Geometry: final body of the model. Coordinates: model frame, mm. Face numbers are marked on the shaded views. Give positions to 0.01 mm unless a question says otherwise; leave off trailing zeros. Write each loop counter-clockwise with the first axis right and the second up, starting at its lowest first coordinate (ties: lowest second). Pieces come first, ordered by that corner, then holes.
Autodesk Inventor part; units mm, degrees
ref_plane "YZ Plane" through (0, 0, 0) normal (1, 0, 0) x (0, 1, 0)
ref_plane "XZ Plane" through (0, 0, 0) normal (0, 1, 0) x (-1, 0, 0)
ref_plane "XY Plane" through (0, 0, 0) normal (0, 0, 1) x (1, 0, 0)
sketch "Эскиз1" plane through (0, 0, 0) normal (0, 0, 1) x (1, 0, 0)
  line L0 (0, 14) -> (0, -14)
  line L1 (21, 14) -> (21.6, 14)
  line L2 (22, 13.6) -> (22, -13.6)
  line L3 (21.6, -14) -> (21, -14)
  line L4 (21, -14) -> (21, 14)
  line L5 (22, 13.6) -> (21.6, 14)
  line L6 (22, -13.6) -> (21.6, -14)
  point P0 (0, 0)
  point P1 (0, 0)
  point P2 (22, -14)
  point P3 (22, 14)
  dimension "d0" = 28
  dimension "d1" = 44
  dimension "d2" = 42
  dimension "d3" = 0.4
  dimension "d4" = 45
  dimension "d5" = 0.4
  dimension "d6" = 45
revolve "Вращение1" add sketch "Эскиз1" angle 360 about axis through (0, 14, 0) along (0, -1, 0)
sketch "Эскиз2" plane through (0, 0, 0) normal (0, 0, 1) x (1, 0, 0)
  circle A0 centre (0, 0) radius 5
  dimension "d8" = 10
extrude "Выдавливание1" cut sketch "Эскиз2" along normal through all both and the other way through all
equation "\"d6\" = d4"
properties part number "75. Втулка шестерни второй передачи"
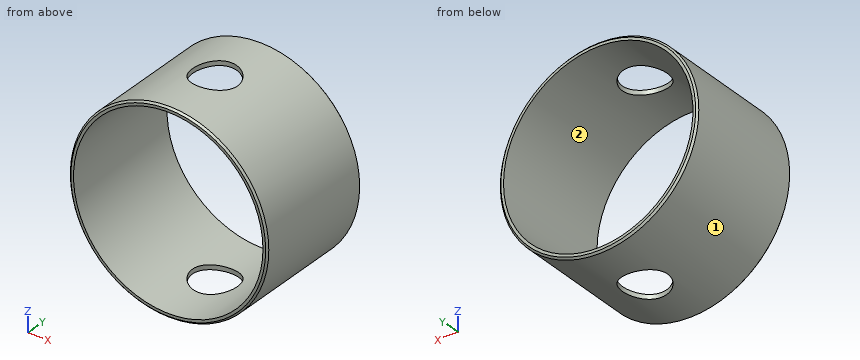
Q1. Section A-A on x = 0. Output: boundary loops of the cut face in (y, z), plus the area to 3 significant figures.
Filled sheet:
outline: (-14, -21.6) - (-13.6, -22) - (-5, -22) - (-5, -21) - (-14, -21) - close; (-14, 21) - (-5, 21) - (-5, 22) - (-13.6, 22) - (-14, 21.6) - close; (5, -22) - (13.6, -22) - (14, -21.6) - (14, -21) - (5, -21) - close; (5, 21) - (14, 21) - (14, 21.6) - (13.6, 22) - (5, 22) - close
area: 35.7 mm2
Q2. Pull-direction query (Z, two-part tool) for the marked faces 1 and 2; classes: released by +Z, released by -Z, zero draft, split by the parting line, or undercut.
Filled sheet:
face 1: split by the parting line
face 2: undercut
Q3. Section D-D on y = 6.5. Output: boundary loops of the cut face in (x, z), plus the area to 3 significant figures.
Filled sheet:
outline: circle Ø44 at (0, 0); hole circle Ø42 at (0, 0)
area: 135 mm2
Q4. Section B-B on z = 0. Output: boundary loops of the cut face in (x, y).
Filled sheet:
outline: (-22, -13.6) - (-21.6, -14) - (-21, -14) - (-21, 14) - (-21.6, 14) - (-22, 13.6) - close; (21, -14) - (21.6, -14) - (22, -13.6) - (22, 13.6) - (21.6, 14) - (21, 14) - close
Q5. Pin query (flat end, axial travel): P1, Ø5, axis at y = 4.5, z = 10, coming from the +X side; P2, Ø3, axis at x = -15, y = -3, coming from the +Z side; P3, Ø6, axis at x = 3.5, y = -3.5, coming from the +Z side. Return the tip coordinate at first contact, or that it passes through.
Filled sheet:
P1: stops at x = 20.68
P2: stops at z = 17.37
P3: stops at z = 21.98
Q6. Ray query, line 1 along Y through (x, z) = (0, 21.2); line 2 along Z through (x, y) = (0, 7.75); line 3 along Z through (x, y) = (17, -6.25). Return the intervals inside material, ascending.
Filled sheet:
line 1: y = -14 to -5, 5 to 14
line 2: z = -22 to -21, 21 to 22
line 3: z = -13.96 to -12.33, 12.33 to 13.96
